from build123d import *

# Parameters (mm, degrees)
BOSS_EXTRUDE3_DEPTH = 5
SKETCH5_R           = 10
BOSS_EXTRUDE4_DEPTH = 60
SKETCH6_R           = 2
CUT_EXTRUDE1_DEPTH  = 20
SKETCH9_W           = 3.11933689
SKETCH9_H           = 7.065160472
CUT_EXTRUDE3_DEPTH  = 60


with BuildPart() as part:
    # Sketch3 → Boss-Extrude3 (new body)
    with BuildSketch(Plane.XY):
        Polygon((6, 10.392304845), (-6, 10.392304845), (-12, 0), (-6, -10.392304845), (6, -10.392304845), (12, 0), align=None)
    extrude(amount=BOSS_EXTRUDE3_DEPTH)

    # Sketch5 → Boss-Extrude4 (add)
    with BuildSketch(Plane.XY.offset(5)):
        Circle(SKETCH5_R)
    extrude(amount=BOSS_EXTRUDE4_DEPTH)

    # Sketch6 → Cut-Extrude1 (cut)
    with BuildSketch(Plane.XY.offset(65)):
        Circle(SKETCH6_R)
    extrude(amount=-CUT_EXTRUDE1_DEPTH, mode=Mode.SUBTRACT)

    # Sketch9 → Cut-Extrude3 (cut)
    with BuildSketch(Plane.XY.offset(65)):
        with Locations((0, 10.532580236)):
            Rectangle(SKETCH9_W, SKETCH9_H)
    extrude(amount=-CUT_EXTRUDE3_DEPTH, mode=Mode.SUBTRACT)


solid = part.part
CAD build for the part. Positions are in the model's coordinates, mm. A direction names the side the tool comes from. Coordinates: 2 decimals unless noted, no trailing zeros. Loops run counter-clockwise (first coordinate to the right, second up) from the corner with the lowest first, then second, coordinate; pieces in that order, holes last. Notation, with made-up numbers: (66, 76) - (89, 76) arc R24 ccw to (89, 104) - close; hole circle Ø5 at (-17, 60.5). An arc over 180 degrees is marked (long way). Use one line per item in the form item = value. Start each with the question number.
1) Flat gauge pins, fed straight in: pin 1 (1.5 mm diameter, centred on y = -6.5, z = 29.5, fed in from -X); pin 2 (1.5 mm diameter, centred on x = -1.5, z = 50, fed in from -Y); pin 3 (6 mm diameter, centred on y = 4.5, z = 34.5, fed in from +X). Where does each tip first touch, or does it go through?
2) Drill centre lines: L1, parallel to Y at x = 0, z = 53.5; L2, parallel to Z at x = 9, y = 4.5; L3, parallel to Z at x = 0.75, y = -1.25. Where is each one in solid material? Low to high. Write a range as from..to.
3) Band-saw the part on B-B (x = 0). Give the cut face in (y, z), and give its area (3 significant figures).
4) Two-plate mould, pull along X, no slides. Class faces 4 (the face through (8.958, -5.269, 2.465)), 5 (the face through (1.56, 8, 35)), 6 (the face through (-9.042, -5.123, 2.465)): +X half, -X half, draft (parallel to the pull), parting line (faces both ways), or undercut.
5) Tool access for faces 1 (the face through (0, -2, 55)), 2 (the face through (0, 7, 35)), 3 (the face through (-8.958, 5.269, 2.465)): list every direction of +Z, -Z, +X, -X, +Y, -Y with a clear straight run to the whole face (end or side of a thin tool).
6) Band-saw the part on D-D (x = -7). Give the cut face in (y, z).
7) Band-saw the part on A-A (z = 46). Give the cut face in (x, y).
8) Band-saw the part on C-C (z = 7.5). Give the cut face in (x, y), and give its area (3 significant figures).
Check values:
q1.pin_1 = -8.18
q1.pin_2 = -9.97
q1.pin_3 = 9.89
q2.L1 = -10..-2, 2..7
q2.L2 = 0..5
q2.L3 = 0..45
q3.outline = (-10.39, 0) - (10.39, 0) - (10.39, 5) - (7, 5) - (7, 65) - (2, 65) - (2, 45) - (-2, 45) - (-2, 65) - (-10, 65) - (-10, 5) - (-10.39, 5) - close
q3.area = 1,040 mm2
q4.face_4 = +X half
q4.face_5 = undercut
q4.face_6 = -X half
q5.face_1 = +Z
q5.face_2 = +Z, +Y
q5.face_3 = +Z, -Z, -X, +Y
q6.outline = (-8.66, 0) - (8.66, 0) - (8.66, 5) - (7.14, 5) - (7.14, 65) - (-7.14, 65) - (-7.14, 5) - (-8.66, 5) - close
q7.outline = (-1.56, 7) - (-1.56, 9.88) arc R10 ccw (long way) to (1.56, 9.88) - (1.56, 7) - close; hole circle Ø4 at (0, 0)
q8.outline = (-1.56, 7) - (-1.56, 9.88) arc R10 ccw (long way) to (1.56, 9.88) - (1.56, 7) - close
q8.area = 305 mm2
